```python
from build123d import *

# Parameters (mm, degrees)
SKETCH_1_R          = 4.25
EXTRUDE_1_DEPTH     = 36.75
SKETCH_2_R          = 3
EXTRUDE_2_DEPTH     = 1
SKETCH_3_R          = 2.5
EXTRUDE_3_DEPTH     = 5
EXTRUDE_START       = 3.5
SKETCH_4_R          = 3
EXTRUDE_4_DEPTH     = 3.5
EXTRUDE_START_2     = 5
SKETCH_5_R          = 2.5
EXTRUDE_5_DEPTH     = 5
CHAMFER_1_SIZE      = 0.5
CHAMFER_2_SIZE      = 0.5
CUT_EXTRUDE_6_REACH = 90.205
SKETCH_6_W          = 6
SKETCH_6_H          = 3
SKETCH_7_R          = 4.25
SKETCH_7_R_2        = 3.25
CUT_EXTRUDE_1_DEPTH = 71.5


with BuildPart() as part:
    # 草图1 → 拉伸1 (new, symmetric)
    with BuildSketch(Plane.XY):
        Circle(SKETCH_1_R)
    extrude(amount=EXTRUDE_1_DEPTH, both=True)

    # 草图2 → 拉伸2 (add)
    with BuildSketch(Plane.XY.offset(36.75)):
        Circle(SKETCH_2_R)
    extrude(amount=EXTRUDE_2_DEPTH)

    # 草图3 → 拉伸3 (add)
    with BuildSketch(Plane.XY.offset(37.75)):
        Circle(SKETCH_3_R)
    extrude(amount=EXTRUDE_3_DEPTH)

    # 草图4 → 拉伸4 (add)
    with BuildSketch(Plane(origin=(0, 0, -36.75), x_dir=(-1, 0, 0), z_dir=(0, 0, -1)).offset(EXTRUDE_START)):
        with Locations(Location((0, 0, 0), (0, 0, 180))):
            Circle(SKETCH_4_R)
    extrude(amount=-EXTRUDE_4_DEPTH)

    # 草图5 → 拉伸5 (add)
    with BuildSketch(Plane(origin=(0, 0, -40.25), x_dir=(-1, 0, 0), z_dir=(0, 0, -1)).offset(EXTRUDE_START_2)):
        with Locations(Location((0, 0, 0), (0, 0, 180))):
            Circle(SKETCH_5_R)
    extrude(amount=-EXTRUDE_5_DEPTH)

    # 倒角1
    chamfer_1_edges = [part.edges().sort_by_distance(p)[0] for p in [
        (-2.5, 0, 42.75),
        (-2.5, 0, -45.25),
    ]]
    chamfer(chamfer_1_edges, length=CHAMFER_1_SIZE)

    # 倒角2
    chamfer_2_edges = [part.edges().sort_by_distance(p)[0] for p in [
        (-3, 0, -40.25),
    ]]
    chamfer(chamfer_2_edges, length=CHAMFER_2_SIZE - 0.0001)  # a hair under: the kernel refuses the full size

    # 拉伸6: up to this face of the body (flat: up to its plane)
    cut_extrude_6_end = Plane(part.part.faces().sort_by_distance((-4.129791847, 0, -36.75))[0])
    # 草图6 → 拉伸6 (cut, up to the picked face)
    with BuildSketch(Plane(origin=(0, 0, -45.25), x_dir=(-1, 0, 0), z_dir=(0, 0, -1)), mode=Mode.PRIVATE) as cut_extrude_6_sk1:
        with Locations((0, 3.5)):
            Rectangle(SKETCH_6_W, SKETCH_6_H)
    cut_extrude_6_tool1 = split(extrude(cut_extrude_6_sk1.sketch, amount=-CUT_EXTRUDE_6_REACH, mode=Mode.PRIVATE), bisect_by=cut_extrude_6_end, keep=Keep.BOTH, mode=Mode.PRIVATE)
    add(cut_extrude_6_tool1.solids().sort_by(Axis((0, 3.5, -45.25), (0, 0, 1)))[0], mode=Mode.SUBTRACT)

    # 草图7 → 切除-拉伸1 (cut)
    with BuildSketch(Plane.XY.offset(36.75)):
        Circle(SKETCH_7_R)
        Circle(SKETCH_7_R_2, mode=Mode.SUBTRACT)
    extrude(amount=-CUT_EXTRUDE_1_DEPTH, mode=Mode.SUBTRACT)


solid = part.part
```
Input: part model. Units: mm. Frame: model coordinates. A direction names the side the tool comes from. Give positions to 0.01 mm unless a question says otherwise; leave off trailing zeros. Write each loop counter-clockwise with the first axis right and the second up, starting at its lowest first coordinate (ties: lowest second). Pieces come first, ordered by that corner, then holes. Notation, with made-up numbers: (70, -25.75) - (104, -25.75) arc R23 cw to (104, -0.75) - close; hole circle Ø10 at (49, 24.5). An arc over 180 degrees is marked (long way). Write item = value, one per line. Start each with the question number.
1. Ray query, L1, parallel to Y at x = -0.25, z = -29.5; L2, parallel to Z at x = 3, y = 0.5; L3, parallel to Z at x = 2, y = -0.25. Return the intervals inside material, ascending.
2. Section query A-A, the plane z = -9. Output: boundary loops of the cut face in (x, y), then the cut area to 3 significant figures.
3. Access query for faces 1 (the flat face through (0, 0, -45.25)), 2 (the flat face through (0, 0, 42.75)), 3 (the cylindrical face through (0, -3, -38)), 4 (the cylindrical face through (-0.54, -2.44, 39.97)), 5 (the flat face through (0, 2, -40)). Directions: +Z, -Z, +X, -X, +Y, -Y. A direction counts if a zero-diameter tool reaches every point of the face in a straight line with its end or side. Return the directions, or none.
4. First-contact query: pin 1 Ø3 at (x, z) = (2, 20) entering from +Y; pin 2 Ø3 at (x, z) = (1.5, 33) entering from -Y; pin 3 Ø2 at (x, z) = (3.5, -31) entering from -Y. Flat tips, straight axial feed; report the tip coordinate or a pass-through.
Check sheet entries:
q1.L1 = -3.24 to 3.24
q1.L2 = -36.75 to 36.75
q1.L3 = -45.23 to 42.73
q2.outline = circle Ø6.5 at (0, 0)
q2.area = 33.2 mm2
q3.face_1 = -Z, +X, -X, +Y, -Y
q3.face_2 = +Z, +X, -X, +Y, -Y
q3.face_3 = -Z
q3.face_4 = +Z
q3.face_5 = -Z, +X, -X, +Y
q4.pin_1 = 3.21
q4.pin_2 = -3.25
q4.pin_3 = -2.08
